from build123d import *

# Parameters (mm, degrees)
SKETCH_1_R      = 2
SKETCH_1_R_2    = 1.5
SKETCH_1_R_3    = 8
EXTRUDE_1_DEPTH = 2


with BuildPart() as part:
    # 草图1 → 凸台-拉伸1 (new body)
    with BuildSketch(Plane(origin=(0, 0, 0), x_dir=(1, 0, 0), z_dir=(0, 1, 0))):
        with BuildLine():
            Line((394.734384308, 186.437991397), (394.734384308, 47.57418904))
            ThreePointArc((394.734384308, 47.57418904), (392.977024848, 43.331548206), (388.734383891, 41.574189041))
            Line((388.734383891, 41.574189041), (280.734383891, 41.574189041))
            ThreePointArc((280.734383891, 41.574189041), (276.491743204, 43.331548353), (274.734383891, 47.57418904))
            Line((274.734383891, 47.57418904), (274.734383891, 186.437990955))
            ThreePointArc((274.734383891, 186.437990955), (274.37476968, 188.483975832), (273.339034487, 190.284705991))
            ThreePointArc((273.339034487, 190.284705991), (334.734382872, 321.574189041), (396.129734602, 190.284707555))
            ThreePointArc((396.129734602, 190.284707555), (395.093998746, 188.483976956), (394.734384308, 186.437991397))
        make_face()
        with Locations(Location((369.73616956, 276.575974709, 0), (0, 0, 270))):
            Circle(SKETCH_1_R, mode=Mode.SUBTRACT)
        with Locations(Location((369.73616956, 206.572403372, 0), (0, 0, 270))):
            Circle(SKETCH_1_R, mode=Mode.SUBTRACT)
        with Locations(Location((299.732598222, 206.572403372, 0), (0, 0, 270))):
            Circle(SKETCH_1_R, mode=Mode.SUBTRACT)
        with Locations(Location((313.734383891, 157.57418904, 0), (0, 0, 270))):
            Circle(SKETCH_1_R_2, mode=Mode.SUBTRACT)
        with Locations(Location((355.734383891, 157.57418904, 0), (0, 0, 270))):
            Circle(SKETCH_1_R_2, mode=Mode.SUBTRACT)
        with Locations(Location((380.234383891, 133.07418904, 0), (0, 0, 270))):
            Circle(SKETCH_1_R_2, mode=Mode.SUBTRACT)
        with Locations(Location((380.234383891, 158.07418904, 0), (0, 0, 270))):
            Circle(SKETCH_1_R_2, mode=Mode.SUBTRACT)
        with Locations(Location((364.734383891, 61.57418904, 0), (0, 0, 270))):
            Circle(SKETCH_1_R_2, mode=Mode.SUBTRACT)
        with Locations(Location((388.734383891, 61.57418904, 0), (0, 0, 270))):
            Circle(SKETCH_1_R_2, mode=Mode.SUBTRACT)
        with Locations(Location((364.734383891, 91.57418904, 0), (0, 0, 270))):
            Circle(SKETCH_1_R_2, mode=Mode.SUBTRACT)
        with Locations(Location((388.734383891, 91.57418904, 0), (0, 0, 270))):
            Circle(SKETCH_1_R_2, mode=Mode.SUBTRACT)
        with Locations(Location((304.734383891, 61.57418904, 0), (0, 0, 270))):
            Circle(SKETCH_1_R_2, mode=Mode.SUBTRACT)
        with Locations(Location((280.734383891, 61.57418904, 0), (0, 0, 270))):
            Circle(SKETCH_1_R_2, mode=Mode.SUBTRACT)
        with Locations(Location((304.734383891, 91.57418904, 0), (0, 0, 270))):
            Circle(SKETCH_1_R_2, mode=Mode.SUBTRACT)
        with Locations(Location((280.734383891, 91.57418904, 0), (0, 0, 270))):
            Circle(SKETCH_1_R_2, mode=Mode.SUBTRACT)
        with Locations(Location((334.734383891, 316.57418904, 0), (0, 0, 270))):
            Circle(SKETCH_1_R_2, mode=Mode.SUBTRACT)
        with Locations(Location((281.701375302, 294.607197629, 0), (0, 0, 270))):
            Circle(SKETCH_1_R_2, mode=Mode.SUBTRACT)
        with Locations(Location((259.734383891, 241.574189041, 0), (0, 0, 270))):
            Circle(SKETCH_1_R_2, mode=Mode.SUBTRACT)
        with Locations(Location((281.701375302, 188.541180451, 0), (0, 0, 270))):
            Circle(SKETCH_1_R_2, mode=Mode.SUBTRACT)
        with Locations(Location((387.76739248, 188.541180451, 0), (0, 0, 270))):
            Circle(SKETCH_1_R_2, mode=Mode.SUBTRACT)
        with Locations(Location((409.734383891, 241.574189041, 0), (0, 0, 270))):
            Circle(SKETCH_1_R_2, mode=Mode.SUBTRACT)
        with Locations(Location((387.76739248, 294.607197629, 0), (0, 0, 270))):
            Circle(SKETCH_1_R_2, mode=Mode.SUBTRACT)
        with Locations(Location((322.734383891, 306.575974709, 0), (0, 0, 270))):
            Circle(SKETCH_1_R_2, mode=Mode.SUBTRACT)
        with Locations(Location((346.734383891, 306.575974709, 0), (0, 0, 270))):
            Circle(SKETCH_1_R_2, mode=Mode.SUBTRACT)
        with Locations(Location((322.734383891, 276.575974709, 0), (0, 0, 270))):
            Circle(SKETCH_1_R_2, mode=Mode.SUBTRACT)
        with Locations(Location((346.734383891, 276.575974709, 0), (0, 0, 270))):
            Circle(SKETCH_1_R_2, mode=Mode.SUBTRACT)
        with Locations(Location((334.734383891, 309.57418904, 0), (0, 0, 270))):
            Circle(SKETCH_1_R_2, mode=Mode.SUBTRACT)
        with Locations(Location((341.734383891, 309.57418904, 0), (0, 0, 270))):
            Circle(SKETCH_1_R_2, mode=Mode.SUBTRACT)
        with Locations(Location((327.734383891, 309.57418904, 0), (0, 0, 270))):
            Circle(SKETCH_1_R_2, mode=Mode.SUBTRACT)
        with Locations(Location((302.217879596, 301.607197629, 0), (0, 0, 270))):
            Circle(SKETCH_1_R_2, mode=Mode.SUBTRACT)
        with Locations(Location((302.217879596, 294.607197629, 0), (0, 0, 270))):
            Circle(SKETCH_1_R_2, mode=Mode.SUBTRACT)
        with Locations(Location((309.217879596, 294.607197629, 0), (0, 0, 270))):
            Circle(SKETCH_1_R_2, mode=Mode.SUBTRACT)
        with Locations(Location((295.217879596, 294.607197629, 0), (0, 0, 270))):
            Circle(SKETCH_1_R_2, mode=Mode.SUBTRACT)
        with Locations(Location((367.250888185, 301.607197629, 0), (0, 0, 270))):
            Circle(SKETCH_1_R_2, mode=Mode.SUBTRACT)
        with Locations(Location((367.250888185, 294.607197629, 0), (0, 0, 270))):
            Circle(SKETCH_1_R_2, mode=Mode.SUBTRACT)
        with Locations(Location((360.250888185, 294.607197629, 0), (0, 0, 270))):
            Circle(SKETCH_1_R_2, mode=Mode.SUBTRACT)
        with Locations(Location((374.250888185, 294.607197629, 0), (0, 0, 270))):
            Circle(SKETCH_1_R_2, mode=Mode.SUBTRACT)
        with Locations(Location((289.234383891, 133.07418904, 0), (0, 0, 270))):
            Circle(SKETCH_1_R_2, mode=Mode.SUBTRACT)
        with Locations(Location((289.234383891, 158.07418904, 0), (0, 0, 270))):
            Circle(SKETCH_1_R_2, mode=Mode.SUBTRACT)
        with Locations(Location((304.734383891, 47.57418904, 0), (0, 0, 270))):
            Circle(SKETCH_1_R_2, mode=Mode.SUBTRACT)
        with Locations(Location((364.734383891, 47.57418904, 0), (0, 0, 270))):
            Circle(SKETCH_1_R_2, mode=Mode.SUBTRACT)
        with Locations(Location((334.734383891, 47.57418904, 0), (0, 0, 270))):
            Circle(SKETCH_1_R_2, mode=Mode.SUBTRACT)
        with Locations(Location((334.734383891, 136.57418904, 0), (0, 0, 270))):
            Circle(SKETCH_1_R_3, mode=Mode.SUBTRACT)
        with Locations(Location((299.732598222, 276.575974709, 0), (0, 0, 270))):
            Circle(SKETCH_1_R, mode=Mode.SUBTRACT)
        with BuildLine():
            Line((354.234383891, 115.57418904), (354.234383891, 89.57418904))
            ThreePointArc((354.234383891, 89.57418904), (355.734383891, 88.07418904), (357.234383891, 89.57418904))
            Line((357.234383891, 89.57418904), (357.234383891, 115.57418904))
            ThreePointArc((357.234383891, 115.57418904), (355.734383891, 117.07418904), (354.234383891, 115.57418904))
        make_face(mode=Mode.SUBTRACT)
        with BuildLine():
            Line((312.234383891, 115.57418904), (312.234383891, 89.57418904))
            ThreePointArc((312.234383891, 89.57418904), (313.734383891, 88.07418904), (315.234383891, 89.57418904))
            Line((315.234383891, 89.57418904), (315.234383891, 115.57418904))
            ThreePointArc((315.234383891, 115.57418904), (313.734383891, 117.07418904), (312.234383891, 115.57418904))
        make_face(mode=Mode.SUBTRACT)
        with BuildLine():
            Line((373.73438389, 46.07418904), (388.734383949, 46.07418904))
            ThreePointArc((388.734383949, 46.07418904), (390.234384308, 47.574188681), (388.734384668, 49.07418904))
            Line((388.734384668, 49.07418904), (373.734383891, 49.07418904))
            ThreePointArc((373.734383891, 49.07418904), (372.234383891, 47.574189041), (373.73438389, 46.07418904))
        make_face(mode=Mode.SUBTRACT)
        with BuildLine():
            Line((295.734383891, 49.07418904), (280.734383933, 49.07418904))
            ThreePointArc((280.734383933, 49.07418904), (279.234383891, 47.574189156), (280.734383701, 46.07418904))
            Line((280.734383701, 46.07418904), (295.734383891, 46.07418904))
            ThreePointArc((295.734383891, 46.07418904), (297.234383891, 47.57418904), (295.734383891, 49.07418904))
        make_face(mode=Mode.SUBTRACT)
        with BuildLine():
            Line((341.23438389, 46.07418904), (355.734383901, 46.07418904))
            ThreePointArc((355.734383901, 46.07418904), (357.234383363, 47.574189579), (355.734382825, 49.07418904))
            Line((355.734382825, 49.07418904), (341.234383891, 49.07418904))
            ThreePointArc((341.234383891, 49.07418904), (339.734383891, 47.574189041), (341.23438389, 46.07418904))
        make_face(mode=Mode.SUBTRACT)
        with BuildLine():
            Line((328.234383891, 49.07418904), (313.734383817, 49.07418904))
            ThreePointArc((313.734383817, 49.07418904), (312.234383891, 47.5741895), (313.734382898, 46.07418904))
            Line((313.734382898, 46.07418904), (328.234383891, 46.07418904))
            ThreePointArc((328.234383891, 46.07418904), (329.734383891, 47.57418904), (328.234383891, 49.07418904))
        make_face(mode=Mode.SUBTRACT)
    extrude(amount=EXTRUDE_1_DEPTH)


solid = part.part
Geometry: final body of the model. Coordinates: model frame, mm. Round coordinates to 2 decimals unless told otherwise and drop trailing zeros. Loops run counter-clockwise (first coordinate to the right, second up) from the corner with the lowest first, then second, coordinate; pieces in that order, holes last. Notation, with made-up numbers: (44, 10) -> (52, 10) arc R31 cw to (52, 43) -> close; hole circle Ø3 at (70, -12.5). An arc over 180 degrees is marked (long way). One line per question, with ' | ' between items. Start each with the question number.
1. Section C-C on z = -289.5. Output: boundary loops of the cut face in (x, y), and give its area (3 significant figures).
2. Contact query for flat-ended pins moving along their axis: pin 1 (2.5 mm diameter, centred on x = 289.23, z = -133.07, fed in from -Y); pin 2 (1 mm diameter, centred on x = 302, y = 0.5, fed in from -Z); pin 3 (1 mm diameter, centred on y = 1.5, z = -103.5, fed in from -X). Output: stop coordinate, or through.
3. Line query: line 1 along X through (y, z) = (0.8, -108); line 2 along Z through (x, y) = (379.5, 0.55); line 3 along Z through (x, y) = (288, 0.7). Output: solid intervals per line, ascending. Write a range as [from, to].
4. Mould query, pull axis Z, two halves, no side actions, for faces 1 (the face through (336, 0, -184)), 2 (the face through (326.925, 0.986, -138.308)), 3 (the face through (393.023, 0.986, -43.378)). Classes: pulls with the +Z half, pulls with the -Z half, needs draft (parallel to the pull), parting line crosses it, or undercut.
5. Section B-B on z = -195.5. Output: boundary loops of the cut face in (x, y).
6. Section A-A on y = 1.4. Count the separate pieces of the cut face and the enclosed holes in it, and give its area (3 significant figures).
Returned:
1) outline: (270.68, 0) -> (398.79, 0) -> (398.79, 2) -> (270.68, 2) -> close | area: 256 mm2
2) pin 1: passes through | pin 2: stops at z = -314.79 | pin 3: stops at x = 274.73
3) line 1: x = [274.73, 312.23], [315.23, 354.23], [357.23, 394.73] | line 2: z = [-307.88, -159.38], [-156.77, -134.38], [-131.77, -49.07], [-46.07, -41.57] | line 3: z = [-306.5, -158.93], [-157.22, -133.93], [-132.22, -49.07], [-46.07, -41.57]
4) face 1: needs draft | face 2: undercut | face 3: pulls with the +Z half
5) outline: (269.33, 0) -> (400.13, 0) -> (400.13, 2) -> (269.33, 2) -> close
6) separate pieces: 1 | enclosed holes: 50 | area: 34,600 mm2
